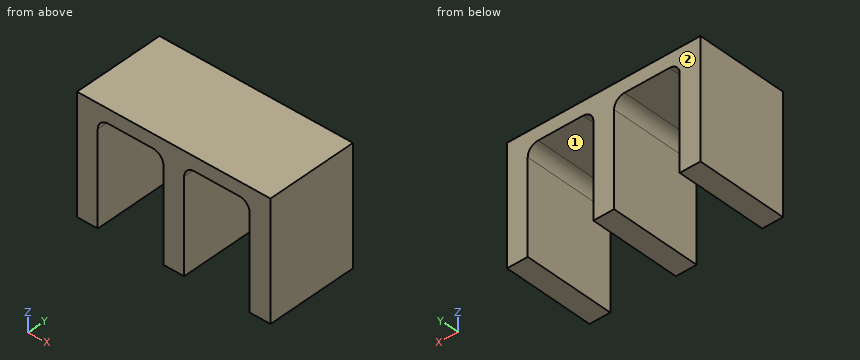
from build123d import *

# Parameters (mm, degrees)
F0_W     = 280
F0_H     = 132
F1_DEPTH = 20
F2_W     = 30
F2_H     = 132
F3_DEPTH = 150
F4_R     = 15
F5_R     = 15


with BuildPart() as f1:
    # F0 (on Top) → F1 (new body)
    with BuildSketch(Plane.XY):
        with Locations((-3.179513, -33.939106)):
            Rectangle(F0_W, F0_H)
    extrude(amount=F1_DEPTH)

    # F2 (on face) → F3 (join)
    with BuildSketch(Plane(origin=(0, 0, 0), x_dir=(1, 0, 0), z_dir=(0, 0, -1))):
        with Locations((121.820487, 33.939106)):
            Rectangle(F2_W, F2_H)
        with Locations((-3.179513, 33.939106)):
            Rectangle(F2_W, F2_H)
        with Locations((-128.179513, 33.939106)):
            Rectangle(F2_W, F2_H)
    extrude(amount=F3_DEPTH)

    # F4
    f4_edges = [f1.edges().sort_by_distance(p)[0] for p in [
        (106.820487, -33.939106, 0),
        (-18.179513, -33.939106, 0),
    ]]
    fillet(f4_edges, radius=F4_R)

    # F5
    f5_edges = [f1.edges().sort_by_distance(p)[0] for p in [
        (-113.179513, -33.939106, 0),
        (11.820487, -33.939106, 0),
    ]]
    fillet(f5_edges, radius=F5_R)


solid = f1.part
Geometry check sheet. Reference: the model listing, model coordinates, mm. Face numbers are marked on the shaded views. A direction names the side the tool comes from. Round coordinates to 2 decimals unless told otherwise and drop trailing zeros. Loops run counter-clockwise (first coordinate to the right, second up) from the corner with the lowest first, then second, coordinate; pieces in that order, holes last.
Item 1: Gauge pin test, flat end, axial feed: pin 1 (19.5 mm diameter, centred on x = -58, y = -41.5, fed in from -Z). Record the tip position at first contact, or that the pin passes through.
Item 2: Cross-section at C-C on x = -37. Record the boundary of the cut face in (y, z).
Item 3: Cross-section at B-B on y = -90. Record the boundary of the cut face in (x, z).
Item 4: Thickness scan on line 1 (X direction, y = -78, z = -37); line 2 (X direction, y = -69, z = -6.5); line 3 (Z direction, x = -74.5, y = -56). Record the ranges inside material, lowest first.
Item 5: Access from +Z, -Z, +X, -X, +Y, -Y to the whole of each face (thin tool, end or side, straight path). Record for the marked faces 1 and 2.
Item 6: Cross-section at A-A on z = -81. Record the boundary of the cut face in (x, y).
Answer sheet:
1. pin 1: stops at z = 0
2. outline: (-99.94, 0) - (32.06, 0) - (32.06, 20) - (-99.94, 20) - close
3. outline: (-143.18, -150) - (-113.18, -150) - (-113.18, -15) arc R15 cw to (-98.18, 0) - (-33.18, 0) arc R15 cw to (-18.18, -15) - (-18.18, -150) - (11.82, -150) - (11.82, -15) arc R15 cw to (26.82, 0) - (91.82, 0) arc R15 cw to (106.82, -15) - (106.82, -150) - (136.82, -150) - (136.82, 20) - (-143.18, 20) - close
4. line 1: x = -143.18 to -113.18, -18.18 to 11.82, 106.82 to 136.82
4. line 2: x = -143.18 to -110.54, -20.82 to 14.46, 104.18 to 136.82
4. line 3: z = 0 to 20
5. face 1: -Z, +Y, -Y
5. face 2: +Z, -Z, +X, -X, +Y
6. outline: (-143.18, -99.94) - (-113.18, -99.94) - (-113.18, 32.06) - (-143.18, 32.06) - close; (-18.18, -99.94) - (11.82, -99.94) - (11.82, 32.06) - (-18.18, 32.06) - close; (106.82, -99.94) - (136.82, -99.94) - (136.82, 32.06) - (106.82, 32.06) - close
